The figure shows three views and two pictorial views of one solid part (mm, origin at its lowest corner). Answer the questions. Round coordinates to 2 decimals unless told otherwise and drop trailing zeros. Loops run counter-clockwise (first coordinate to the right, second up) from the corner with the lowest first, then second, coordinate; pieces in that order, holes last. Notation, with made-up numbers: (4, -9.5) -> (14, -9.5) arc R18 ccw to (14, 18.5) -> close; hole circle Ø1 at (-38, -13.5). An arc over 180 degrees is marked (long way). Put each result on its own line as item: value.
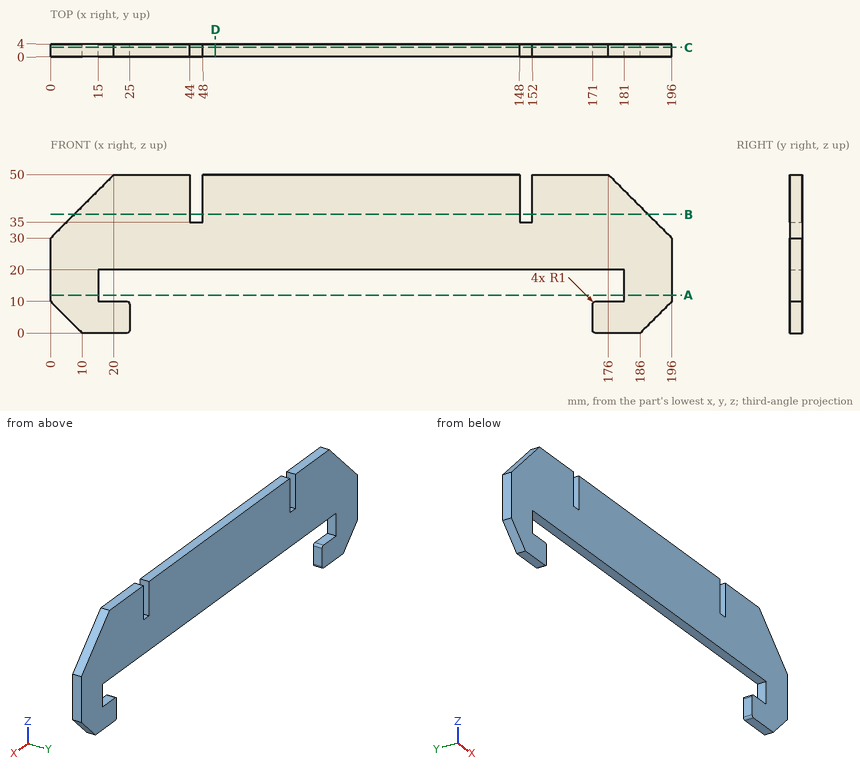
Item 1: Find the intervals of material crossed by line 1 along X through (y, z) = (0.4, 38.5); line 2 along X through (y, z) = (3.75, 37.5); line 3 along Z through (x, y) = (18, 2), in increasing order.
Derived:
line 1: x = 8.5 to 44, 48 to 148, 152 to 187.5
line 2: x = 7.5 to 44, 48 to 148, 152 to 188.5
line 3: z = 0 to 10, 20 to 48
Item 2: The part is cut by section B-B (z = 37.5). Determine the outline of the cut face in (x, y), then the cut area to 3 significant figures.
Derived:
outline: (7.5, 0) -> (44, 0) -> (44, 4) -> (7.5, 4) -> close; (48, 0) -> (148, 0) -> (148, 4) -> (48, 4) -> close; (152, 0) -> (188.5, 0) -> (188.5, 4) -> (152, 4) -> close
area: 692 mm^2
Item 3: The part is cut by section C-C (y = 2.9). Determine the outline of the cut face in (x, z).
Derived:
outline: (0, 10) -> (10, 0) -> (24, 0) arc R1 ccw to (25, 1) -> (25, 9) arc R1 ccw to (24, 10) -> (15, 10) -> (15, 20) -> (181, 20) -> (181, 10) -> (172, 10) arc R1 ccw to (171, 9) -> (171, 1) arc R1 ccw to (172, 0) -> (186, 0) -> (196, 10) -> (196, 30) -> (176, 50) -> (152, 50) -> (152, 35) -> (148, 35) -> (148, 50) -> (48, 50) -> (48, 35) -> (44, 35) -> (44, 50) -> (20, 50) -> (0, 30) -> close
Item 4: The part is cut by section D-D (x = 52). Determine the outline of the cut face in (y, z), then the cut area to 3 significant figures.
Derived:
outline: (0, 20) -> (4, 20) -> (4, 50) -> (0, 50) -> close
area: 120 mm^2
Item 5: Flat-ended cylindrical pins translate along their axes: pin 1 Ø2 at (y, z) = (2.5, 41.5) entering from -X; pin 2 Ø2 at (y, z) = (2.5, 42.5) entering from +X; pin 3 Ø2 at (y, z) = (1.5, 4) entering from +X. Find the tip coordinate at first contact, or state that the pin passes through.
Derived:
pin 1: stops at x = 10.5
pin 2: stops at x = 184.5
pin 3: stops at x = 191
Item 6: The part is cut by section A-A (z = 12). Determine the outline of the cut face in (x, y).
Derived:
outline: (0, 0) -> (15, 0) -> (15, 4) -> (0, 4) -> close; (181, 0) -> (196, 0) -> (196, 4) -> (181, 4) -> close
